from build123d import *

# Parameters (mm, degrees)
SKETCH_1_R          = 2
SKETCH_1_R_2        = 1
EXTRUDE_1_DEPTH     = 28
SKETCH_2_R          = 3
SKETCH_2_R_2        = 2
EXTRUDE_2_DEPTH     = 2.5
EXTRUDE_START       = 25.5
SKETCH_3_R          = 3
SKETCH_3_R_2        = 2
EXTRUDE_3_DEPTH     = 2.5
SKETCH_4_R          = 1.6
CUT_EXTRUDE_1_DEPTH = 1.5
CUT_EXTRUDE_START   = 28
CUT_EXTRUDE_2_DEPTH = 1.6


with BuildPart() as part:
    # 草图1 → 凸台-拉伸1 (new body)
    with BuildSketch(Plane(origin=(0, 0, 0), x_dir=(1, 0, 0), z_dir=(0, 1, 0))):
        with Locations(Location((0, 0, 0), (0, 0, 270))):
            Circle(SKETCH_1_R)
        with Locations(Location((0, 0, 0), (0, 0, 270))):
            Circle(SKETCH_1_R_2, mode=Mode.SUBTRACT)
    extrude(amount=EXTRUDE_1_DEPTH)

    # 草图2 → 凸台-拉伸2 (add)
    with BuildSketch(Plane(origin=(0, 0, 0), x_dir=(1, 0, 0), z_dir=(0, 1, 0))):
        with Locations(Location((0, 0, 0), (0, 0, 270))):
            Circle(SKETCH_2_R)
        with Locations(Location((0, 0, 0), (0, 0, 270))):
            Circle(SKETCH_2_R_2, mode=Mode.SUBTRACT)
    extrude(amount=EXTRUDE_2_DEPTH)

    # 草图3 → 凸台-拉伸3 (add)
    with BuildSketch(Plane(origin=(0, 0, 0), x_dir=(1, 0, 0), z_dir=(0, 1, 0)).offset(EXTRUDE_START)):
        with Locations(Location((0, 0, 0), (0, 0, 270))):
            Circle(SKETCH_3_R)
        with Locations(Location((0, 0, 0), (0, 0, 270))):
            Circle(SKETCH_3_R_2, mode=Mode.SUBTRACT)
    extrude(amount=EXTRUDE_3_DEPTH)

    # 草图4 → 切除-拉伸1 (cut)
    with BuildSketch(Plane(origin=(0, 0, 0), x_dir=(1, 0, 0), z_dir=(0, 1, 0))):
        with Locations(Location((0, 0, 0), (0, 0, 270))):
            Circle(SKETCH_4_R)
    extrude(amount=CUT_EXTRUDE_1_DEPTH, mode=Mode.SUBTRACT)

    # 草图5 → 切除-拉伸2 (cut)
    with BuildSketch(Plane(origin=(0, 0, 0), x_dir=(1, 0, 0), z_dir=(0, 1, 0)).offset(CUT_EXTRUDE_START)):
        Polygon((0, -2.309401077), (2, -1.154700538), (2, 1.154700538), (0, 2.309401077), (-2, 1.154700538), (-2, -1.154700538), align=None)
    extrude(amount=-CUT_EXTRUDE_2_DEPTH, mode=Mode.SUBTRACT)


solid = part.part
Read the model definition and answer for the solid it produces. Units are mm, in the model's axes. A direction names the side the tool comes from. Give positions to 0.01 mm unless a question says otherwise; leave off trailing zeros. Loops run counter-clockwise (first coordinate to the right, second up) from the corner with the lowest first, then second, coordinate; pieces in that order, holes last. Notation, with made-up numbers: (73.25, 28) -> (111.25, 28) arc R23 cw to (111.25, 50) -> close; hole circle Ø9 at (-10.5, -27.75). An arc over 180 degrees is marked (long way). Use a Markdown table: item, result.
Q1. Each of these flat-tipped pins is pushed along its axis until it touches: pin 1 (1 mm diameter, centred on x = -2, y = 3.5, fed in from -Z); pin 2 (3 mm diameter, centred on x = 1.5, y = 8.5, fed in from -Z); pin 3 (3 mm diameter, centred on y = 12, z = 0.5, fed in from -X). Where does it stop, or does it pass through?
Solved:
| item | result |
|---|---|
| pin 1 | stops at z = -1.32 |
| pin 2 | stops at z = -2 |
| pin 3 | stops at x = -2 |
Q2. Section C-C, the plane y = 15.5 is taken. Determine the outline of the cut face in (x, z), then the cut area to 3 significant figures.
Solved:
| item | result |
|---|---|
| outline | circle Ø4 at (0, 0); hole circle Ø2 at (0, 0) |
| area | 9.42 mm^2 |
Q3. Find the intervals of material crossed by line 1 along X through (y, z) = (1, 0); line 2 along X through (y, z) = (11.75, 0); line 3 along Z through (x, y) = (-0.1, 21), in increasing order.
Solved:
| item | result |
|---|---|
| line 1 | x = -3 to -1.6, 1.6 to 3 |
| line 2 | x = -2 to -1, 1 to 2 |
| line 3 | z = -2 to -0.99, 0.99 to 2 |
Q4. Determine the mould class of faces 1 (the face through (0.9, 1.23, 2.86)), 2 (the face through (-2, 27, 0)), 3 (the face through (-1, 25.5, 2)) for opening direction X: pulls with the +X half, pulls with the -X half, needs draft (parallel to the pull), parting line crosses it, or undercut.
Solved:
| item | result |
|---|---|
| face 1 | parting line crosses it |
| face 2 | undercut |
| face 3 | needs draft |
Q5. A tool of negligible diameter and unlimited length cuts with its end or side. For faces 4 (the face through (-0.97, 0.74, -1.27)), 5 (the face through (0.9, 26.73, 2.86)), 6 (the face through (-1, 26.4, -1)), 7 (the face through (-2, 14, 0)), from which of +Z, -Z, +X, -X, +Y, -Y can it reach the whole face along a straight path? Write none if from no direction.
Solved:
| item | result |
|---|---|
| face 4 | -Y |
| face 5 | +Y, -Y |
| face 6 | +Y |
| face 7 | none |
Q6. Section B-B, the plane x = 2.35 is taken. Determine the outline of the cut face in (y, z).
Solved:
| item | result |
|---|---|
| outline | (0, -1.86) -> (2.5, -1.86) -> (2.5, 1.86) -> (0, 1.86) -> close; (25.5, -1.86) -> (28, -1.86) -> (28, 1.86) -> (25.5, 1.86) -> close |
Q7. Section A-A, the plane z = 0 is taken. Determine the outline of the cut face in (x, y).
Solved:
| item | result |
|---|---|
| outline | (-3, 0) -> (-1.6, 0) -> (-1.6, 1.5) -> (-1, 1.5) -> (-1, 26.4) -> (-2, 26.4) -> (-2, 28) -> (-3, 28) -> (-3, 25.5) -> (-2, 25.5) -> (-2, 2.5) -> (-3, 2.5) -> close; (1, 1.5) -> (1.6, 1.5) -> (1.6, 0) -> (3, 0) -> (3, 2.5) -> (2, 2.5) -> (2, 25.5) -> (3, 25.5) -> (3, 28) -> (2, 28) -> (2, 26.4) -> (1, 26.4) -> close |
